from build123d import *

# Parameters (mm, degrees)
BOSS_EXTRUDE1_DEPTH = 12.7
SKETCH2_R           = 1.5875
CUT_EXTRUDE1_DEPTH  = 67.009021317
FILLET5_R           = 6.35
FILLET6_R           = 3.175
CHAMFER1_START      = -12.7
CHAMFER1_DEPTH      = 25.4
CHAMFER1_2_DEPTH    = 5.842
CHAMFER1_START_2    = 37.918945752
CHAMFER1_3_DEPTH    = 5.842
CUT_EXTRUDE2_REACH  = 62.01
SKETCH4_W           = 12.7
SKETCH4_H           = 1.5875


with BuildPart() as part:
    # Sketch1 → Boss-Extrude1 (new body)
    with BuildSketch(Plane(origin=(0, 0, 0), x_dir=(1, 0, 0), z_dir=(0, 1, 0))):
        Polygon((0, 9.525), (-12.7, 9.525), (-12.7, 15.875), (6.35, 15.875), (6.35, 6.35), (37.410945752, 6.35), (37.410945752, 15.875), (56.460945752, 15.875), (56.460945752, 9.525), (43.760945752, 9.525), (43.760945752, -9.525), (56.460945752, -9.525), (56.460945752, -15.875), (37.410945752, -15.875), (37.410945752, -6.35), (6.35, -6.35), (6.35, -15.875), (-12.7, -15.875), (-12.7, -9.525), (0, -9.525), align=None)
    extrude(amount=BOSS_EXTRUDE1_DEPTH)

    # Sketch2 → Cut-Extrude1 (cut, through all)
    with BuildSketch(Plane.XY.offset(15.875)):
        with Locations((50.110945752, 6.35)):
            Circle(SKETCH2_R)
        with Locations((-6.35, 6.35)):
            Circle(SKETCH2_R)
    extrude(amount=-CUT_EXTRUDE1_DEPTH, mode=Mode.SUBTRACT)

    # Fillet5
    fillet5_edges = [part.edges().sort_by_distance(p)[0] for p in [
        (56.460945752, 0, 12.7),
        (56.460945752, 12.7, 12.7),
        (56.460945752, 0, -12.7),
        (56.460945752, 12.7, -12.7),
        (-12.7, 12.7, 12.7),
        (-12.7, 0, 12.7),
        (-12.7, 0, -12.7),
        (-12.7, 12.7, -12.7),
    ]]
    fillet(fillet5_edges, radius=FILLET5_R - 0.0001)  # a hair under: the kernel refuses the full size

    # Fillet6
    fillet6_edges = [part.edges().sort_by_distance(p)[0] for p in [
        (43.760995752, 0, 15.875),
        (54.601103102, 1.85984265, 15.875),
        (54.601103102, 10.84015735, 15.875),
        (43.760995752, 0, -15.875),
        (54.601103102, 1.85984265, -15.875),
        (54.601103102, 10.84015735, -15.875),
        (-5e-05, 0, -15.875),
        (-10.84015735, 1.85984265, -15.875),
        (-10.84015735, 10.84015735, -15.875),
        (-5e-05, 12.7, 15.875),
        (-5e-05, 0, 15.875),
        (-10.84015735, 1.85984265, 15.875),
        (-3.17505, 12.7, -9.525),
        (-3.17505, 0, -9.525),
        (-10.84015735, 1.85984265, -9.525),
        (-3.17505, 0, 9.525),
        (-10.84015735, 1.85984265, 9.525),
        (-3.17505, 12.7, 9.525),
        (46.935995752, 0, -9.525),
        (54.601103102, 1.85984265, -9.525),
        (46.935995752, 12.7, -9.525),
        (46.935995752, 12.7, 9.525),
        (46.935995752, 0, 9.525),
        (54.601103102, 1.85984265, 9.525),
        (43.760995752, 12.7, 15.875),
        (43.760995752, 12.7, -15.875),
        (-5e-05, 12.7, -15.875),
        (-10.84015735, 10.84015735, 15.875),
        (-10.84015735, 10.84015735, -9.525),
        (-10.84015735, 10.84015735, 9.525),
        (54.601103102, 10.84015735, -9.525),
        (54.601103102, 10.84015735, 9.525),
    ]]
    fillet(fillet6_edges, radius=FILLET6_R - 0.0001)  # a hair under: the kernel refuses the full size

    # Chamfer1: read off the stored shape, not the designer's step
    # Chamfer1 outline → Chamfer1 (cut)
    with BuildSketch(Plane.XY.offset(CHAMFER1_START)):
        Polygon((43.760945752, 5.842), (37.918945752, 0), (43.760945752, 0), align=None)
        Polygon((0, 0), (5.842, 0), (0, 5.842), align=None)
        Polygon((37.918945752, 12.7), (43.760945752, 6.858), (43.760945752, 12.7), align=None)
        Polygon((0, 12.7), (0, 6.858), (5.842, 12.7), align=None)
    extrude(amount=CHAMFER1_DEPTH, mode=Mode.SUBTRACT)

    # Chamfer1 2 outline → Chamfer1 2 (add)
    with BuildSketch(Plane.YZ):
        with BuildLine():
            Line((6.858, 9.525), (9.525, 9.525))
            ThreePointArc((9.525, 9.525), (11.77006403, 10.45493597), (12.7, 12.7))
            Line((12.7, 12.7), (6.858, 12.7))
            Line((6.858, 12.7), (6.858, 9.525))
        make_face()
        with BuildLine():
            ThreePointArc((3.175, -9.525), (0.92993597, -10.45493597), (0, -12.7))
            Line((0, -12.7), (5.842, -12.7))
            Line((5.842, -12.7), (5.842, -9.525))
            Line((5.842, -9.525), (3.175, -9.525))
        make_face()
        with BuildLine():
            Line((6.858, -9.525), (6.858, -12.7))
            Line((6.858, -12.7), (12.7, -12.7))
            ThreePointArc((12.7, -12.7), (11.77006403, -10.45493597), (9.525, -9.525))
            Line((9.525, -9.525), (6.858, -9.525))
        make_face()
        with BuildLine():
            ThreePointArc((0, 12.7), (0.92993597, 10.45493597), (3.175, 9.525))
            Line((3.175, 9.525), (5.842, 9.525))
            Line((5.842, 9.525), (5.842, 12.7))
            Line((5.842, 12.7), (0, 12.7))
        make_face()
    extrude(amount=CHAMFER1_2_DEPTH)

    # Chamfer1 3 outline → Chamfer1 3 (add)
    with BuildSketch(Plane.YZ.offset(CHAMFER1_START_2)):
        with BuildLine():
            Line((6.858, 9.525), (9.525, 9.525))
            ThreePointArc((9.525, 9.525), (11.77006403, 10.45493597), (12.7, 12.7))
            Line((12.7, 12.7), (6.858, 12.7))
            Line((6.858, 12.7), (6.858, 9.525))
        make_face()
        with BuildLine():
            ThreePointArc((3.175, -9.525), (0.92993597, -10.45493597), (0, -12.7))
            Line((0, -12.7), (5.842, -12.7))
            Line((5.842, -12.7), (5.842, -9.525))
            Line((5.842, -9.525), (3.175, -9.525))
        make_face()
        with BuildLine():
            Line((6.858, -9.525), (6.858, -12.7))
            Line((6.858, -12.7), (12.7, -12.7))
            ThreePointArc((12.7, -12.7), (11.77006403, -10.45493597), (9.525, -9.525))
            Line((9.525, -9.525), (6.858, -9.525))
        make_face()
        with BuildLine():
            ThreePointArc((0, 12.7), (0.92993597, 10.45493597), (3.175, 9.525))
            Line((3.175, 9.525), (5.842, 9.525))
            Line((5.842, 9.525), (5.842, 12.7))
            Line((5.842, 12.7), (0, 12.7))
        make_face()
    extrude(amount=CHAMFER1_3_DEPTH)

    # Cut-Extrude2: up to this plane
    cut_extrude2_end = Plane(origin=(5.842, 12.7, 0), z_dir=(0.7071067811865497, -0.7071067811865455, 0))
    # Sketch4 → Cut-Extrude2 (cut, up to the surface)
    with BuildSketch(Plane(origin=(43.760945752, 0, 0), x_dir=(0, 0, -1), z_dir=(1, 0, 0)), mode=Mode.PRIVATE) as cut_extrude2_sk1:
        with Locations((0, 11.90625)):
            Rectangle(SKETCH4_W, SKETCH4_H)
    cut_extrude2_tool1 = split(extrude(cut_extrude2_sk1.sketch, amount=-CUT_EXTRUDE2_REACH, mode=Mode.PRIVATE), bisect_by=cut_extrude2_end, keep=Keep.BOTH, mode=Mode.PRIVATE)
    add(cut_extrude2_tool1.solids().sort_by_distance((43.760946, 11.90625, 0))[0], mode=Mode.SUBTRACT)
    # Sketch4 → Cut-Extrude2 (cut, up to the surface)
    with BuildSketch(Plane(origin=(43.760945752, 0, 0), x_dir=(0, 0, -1), z_dir=(1, 0, 0)), mode=Mode.PRIVATE) as cut_extrude2_sk2:
        with Locations((0, 0.79375)):
            Rectangle(SKETCH4_W, SKETCH4_H)
    cut_extrude2_tool2 = split(extrude(cut_extrude2_sk2.sketch, amount=-CUT_EXTRUDE2_REACH, mode=Mode.PRIVATE), bisect_by=cut_extrude2_end, keep=Keep.BOTH, mode=Mode.PRIVATE)
    add(cut_extrude2_tool2.solids().sort_by_distance((43.760946, 0.79375, 0))[0], mode=Mode.SUBTRACT)


solid = part.part
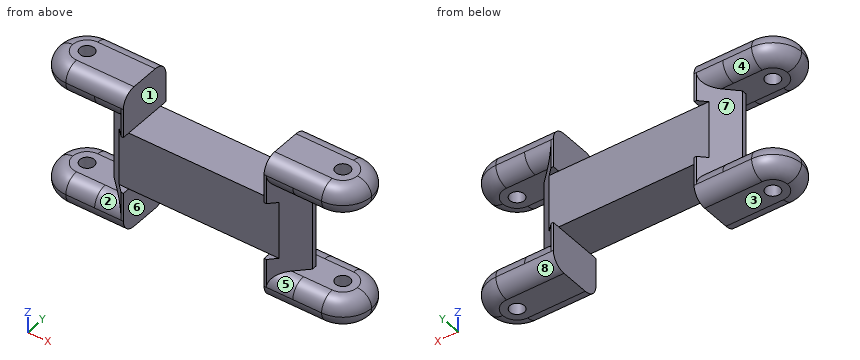
Read the model definition and answer for the solid it produces. Units are mm, in the model's axes. Face numbers are marked on the shaded views. A direction names the side the tool comes from. Round coordinates to 2 decimals unless told otherwise and drop trailing zeros. Write each loop counter-clockwise with the first axis right and the second up, starting at its lowest first coordinate (ties: lowest second). Pieces come first, ordered by that corner, then holes. Notation, with made-up numbers: (-11.5, 12) - (24.5, 12) arc R18 cw to (24.5, 25) - close; hole circle Ø2 at (-31, 44). An arc over 180 degrees is marked (long way). Use a Markdown table: item, result.
(1) The part is cut by section A-A (z = 2.5). Write down the section's boundary in (x, y), then the cut area to 3 significant figures.
Reported:
| item | result |
|---|---|
| outline | (0, 5.84) - (4.25, 1.59) - (39.51, 1.59) - (43.76, 5.84) - (43.76, 6.86) - (39.51, 11.11) - (4.25, 11.11) - (0, 6.86) - close |
| area | 381 mm2 |
(2) Each of these flat-tipped pins is pushed along its axis until it touches: pin 1 Ø5 at (x, y) = (16, 8) entering from -Z; pin 2 Ø0.5 at (x, y) = (5, 0.5) entering from -Z; pin 3 Ø5 at (y, z) = (3.5, -12.5) entering from -X. Where does it stop, or does it pass through?
Reported:
| item | result |
|---|---|
| pin 1 | z = -6.35 |
| pin 2 | z = -14.75 |
| pin 3 | x = -12.69 |
(3) The part is cut by section C-C (x = 30). Write down the section's boundary in (y, z), then the cut area to 3 significant figures.
Reported:
| item | result |
|---|---|
| outline | (1.59, -6.35) - (11.11, -6.35) - (11.11, 6.35) - (1.59, 6.35) - close |
| area | 121 mm2 |
(4) Straight lines are drawn through the part: line 1 along Y through (x, z) = (-6.35, 12.5); line 2 along Z through (x, y) = (-2, 6) (3 decimals); line 3 along Z through (x, y) = (21.5, 10.5). For each, find the intervals that lie inside material, in ascending order. Write a range as [from, to].
Reported:
| item | result |
|---|---|
| line 1 | [0.01, 4.76], [7.94, 12.69] |
| line 2 | [-15.875, -9.525], [9.525, 15.875] |
| line 3 | [-6.35, 6.35] |
(5) Which of the six approach directions +Z, -Z, +X, -X, +Y, -Y give full straight-line access (tool end or side, diameter ignored) to the marked faces 1, 2, 3, 4 and 5?
Reported:
| item | result |
|---|---|
| face 1 | +Z, +Y, -Y |
| face 2 | -X, -Y |
| face 3 | -Z, +X, -X, +Y, -Y |
| face 4 | -X, +Y |
| face 5 | +X, -Y |
(6) The mould has two halves that part along X. Classify the marked faces 6, 7 and 8: released by +X, released by -X, zero draft, split by the parting line, or undercut.
Reported:
| item | result |
|---|---|
| face 6 | undercut |
| face 7 | released by -X |
| face 8 | zero draft |
